Part model, mm, in its own coordinate system. Face numbers are marked on the shaded views. A direction names the side the tool comes from. Round coordinates to 2 decimals unless told otherwise and drop trailing zeros. Loops run counter-clockwise (first coordinate to the right, second up) from the corner with the lowest first, then second, coordinate; pieces in that order, holes last. Notation, with made-up numbers: M 61,29.25 L 88,29.25 A25 cw 88,65.25 Z; hole C 71.25,59.25 d3. An arc over 180 degrees is marked long. Answer as CSV lines item,"result". Start each with the question number.
Item 1: Mould opens along X. For the marked faces 1, 2 and 3 say: pulls with the +X half, pulls with the -X half, needs draft (parallel to the pull), parting line crosses it, or undercut.
Item 2: Band-saw the part on B-B (x = 10.25). Give the cut face in (y, z), and give its area (3 significant figures).
Item 3: Band-saw the part on A-A (y = -5). Give the cut face in (x, z).
Item 4: Which spindle directions (+Z, -Z, +X, -X, +Y, -Y) get a long thin tool onto all of the face, cutting with end or side? Do the marked faces 4 and 5. Say none if no direction does.
Item 5: Wall check: line 1 (X direction, y = -3, z = 11); line 2 (Z direction, x = 12.75, y = -2.75); line 3 (Z direction, x = 7.5, y = -5.25). Give the ranges that are in metal, low to high.
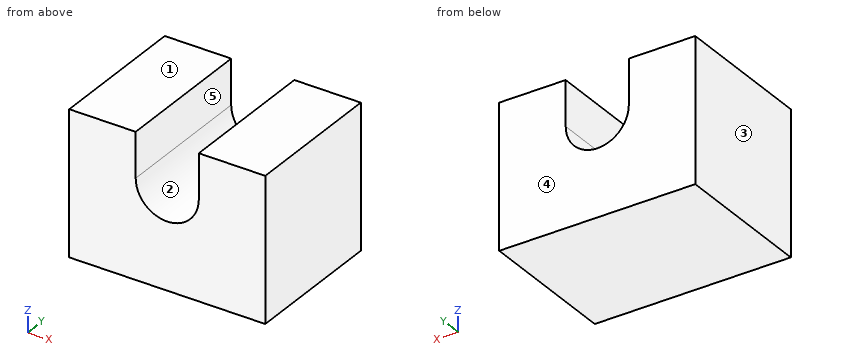
```python
from build123d import *

# Parameters (mm, degrees)
F0_W     = 20.5
F0_H     = 15
F1_DEPTH = 15
F3_DEPTH = 15.001


with BuildPart() as f1:
    # F0 (on Front) → F1 (new body)
    with BuildSketch(Plane.XZ):
        with Locations((10.25, 7.5)):
            Rectangle(F0_W, F0_H)
    extrude(amount=F1_DEPTH)

    # F2 (on face) → F3 (cut, through all)
    with BuildSketch(Plane.XZ.offset(15)):
        with BuildLine():
            ThreePointArc((6.950002, 10.303269), (10.248365, 7), (13.55, 10.3))
            ThreePointArc((13.55, 10.3), (10.251635, 13.6), (6.950002, 10.303269))
        make_face()
        with BuildLine():
            ThreePointArc((6.950002, 10.303269), (10.251635, 13.6), (13.55, 10.3))
            Line((13.55, 10.3), (13.55, 15))
            Line((13.55, 15), (6.950002, 15))
            Line((6.950002, 15), (6.950002, 10.303269))
        make_face()
    extrude(amount=-F3_DEPTH, mode=Mode.SUBTRACT)


solid = f1.part
```
Answer block:
1,face 1,"needs draft"
1,face 2,"undercut"
1,face 3,"pulls with the -X half"
2,outline,"M -15,0 L 0,0 L 0,7 L -15,7 Z"
2,area,"105 mm^2"
3,outline,"M 0,0 L 20.5,0 L 20.5,15 L 13.55,15 L 13.55,10.3 A3.3 cw 6.95,10.3 L 6.95,15 L 0,15 Z"
4,face 4,"+Z, -Z, +X, -X, +Y"
4,face 5,"+Z, +Y, -Y"
5,line 1,"x = 0 to 6.95, 13.55 to 20.5"
5,line 2,"z = 0 to 8.15"
5,line 3,"z = 0 to 8.48"
